```python
from build123d import *

# Parameters (mm, degrees)
SKETCH1_R               = 22.45
BOSS_EXTRUDE1_DEPTH     = 5
SKETCH2_R               = 5
CUT_EXTRUDE1_DEPTH      = 5
BOSS_EXTRUDE2_DEPTH     = 50
BOSS_EXTRUDE5_DEPTH     = 50
CUT_EXTRUDE3_DEPTH      = 64.505944604
CUT_EXTRUDE3_DEPTH_BACK = 64.505944604


with BuildPart() as part:
    # Sketch1 → Boss-Extrude1 (new body)
    with BuildSketch(Plane.XY):
        Circle(SKETCH1_R)
    extrude(amount=BOSS_EXTRUDE1_DEPTH)

    # Sketch2 → Cut-Extrude1 (cut)
    with BuildSketch(Plane(origin=(0, 0, 0), x_dir=(-1, 0, 0), z_dir=(0, 0, -1))):
        Circle(SKETCH2_R)
        with Locations((0, 15)):
            Circle(SKETCH2_R)
    extrude(amount=-CUT_EXTRUDE1_DEPTH, mode=Mode.SUBTRACT)

    # Sketch3 → Boss-Extrude2 (add)
    with BuildSketch(Plane.XY.offset(5)):
        with BuildLine():
            Line((-12.718195627, -18.5), (12.718195627, -18.5))
            ThreePointArc((12.718195627, -18.5), (14.006550731, -17.544772344), (15.223419458, -16.5))
            Line((15.223419458, -16.5), (-15.223419458, -16.5))
            ThreePointArc((-15.223419458, -16.5), (-14.006550731, -17.544772344), (-12.718195627, -18.5))
        make_face()
    extrude(amount=BOSS_EXTRUDE2_DEPTH)

    # Sketch5 → Boss-Extrude5 (add)
    with BuildSketch(Plane.XY.offset(5)):
        with BuildLine():
            Line((-15.223419458, -16.5), (-12.08108025, -16.5))
            ThreePointArc((-12.08108025, -16.5), (-12.994947259, -15.790308602), (-13.867212825, -15.030066815))
            ThreePointArc((-13.867212825, -15.030066815), (-18.732151535, -8.204206169), (-20.45, 0))
            Line((-20.45, 0), (-22.45, 0))
            ThreePointArc((-22.45, 0), (-20.564146795, -9.006573521), (-15.223419458, -16.5))
        make_face()
        with BuildLine():
            Line((20.45, 0), (22.45, 0))
            ThreePointArc((22.45, 0), (20.564146795, -9.006573521), (15.223419458, -16.5))
            Line((15.223419458, -16.5), (12.08108025, -16.5))
            ThreePointArc((12.08108025, -16.5), (12.994947259, -15.790308602), (13.867212825, -15.030066815))
            ThreePointArc((13.867212825, -15.030066815), (18.732151535, -8.204206169), (20.45, 0))
        make_face()
    extrude(amount=BOSS_EXTRUDE5_DEPTH)

    # Sketch6 → Cut-Extrude3 (cut, two sides: drawn at the far end of the back side and taken through both)
    with BuildSketch(Plane(origin=(0, 0, 0), x_dir=(1, 0, 0), z_dir=(0, 1, 0)).offset(-CUT_EXTRUDE3_DEPTH_BACK)):
        Polygon((-22.45, 0), (22.45, 0), (22.45, -2.35310929), align=None)
    extrude(amount=CUT_EXTRUDE3_DEPTH + CUT_EXTRUDE3_DEPTH_BACK, mode=Mode.SUBTRACT)


solid = part.part
```
Source: CAD feature listing. Evaluate the final solid. Frame: model axes, mm. A direction names the side the tool comes from. Give positions to 0.01 mm unless a question says otherwise; leave off trailing zeros. Loops run counter-clockwise (first coordinate to the right, second up) from the corner with the lowest first, then second, coordinate; pieces in that order, holes last. Notation, with made-up numbers: (38, -17.75) - (86, -17.75) arc R9 cw to (86, -10.75) - close; hole circle Ø7 at (2, 34). An arc over 180 degrees is marked (long way). Use CSV: the item, a comma, the result in double quotes. Start each with the question number.
1. Section D-D (y = 4). Output: boundary loops of the cut face in (x, z), then the cut area to 3 significant figures.
2. Reachability of faces 5 (the flat face through (0, -18.5, 30)), 6 (the flat face through (0.314, -5.303, 1.193)), 7 (the flat face through (5, 3, 5)), 8 (the flat face through (-21, 0, 30)) from +Z, -Z, +X, -X, +Y, -Y: full face, straight path, thin tool, end or side. Return the list, or none.
3. Draft query along Y for faces 1 (the flat face through (0, -20, 5)), 2 (the cylindrical face through (-4.619, -1.915, 2.929)), 3 (the flat face through (0, -16.5, 30)), 4 (the cylindrical face through (-4.619, 13.085, 2.929)). Return one class per face: +Y half, -Y half, draft (parallel to the pull), parting line (faces both ways), or undercut.
4. Ray query, L1, parallel to Y at x = 0, z = 3; L2, parallel to X at y = -7, z = 37.5; L3, parallel to X at y = 15, z = 2.5. Return the intervals inside material, ascending.
5. Section C-C (z = 31). Output: boundary loops of the cut face in (x, y), then the cut area to 3 significant figures.
6. Section B-B (x = 3.5). Output: boundary loops of the cut face in (y, z), then the cut area to 3 significant figures.
7. Section A-A (y = -4). Output: boundary loops of the cut face in (x, z).
8. Pin query (flat end, axial travel): pin 1 (3 mm diameter, centred on y = -11.5, z = 14, fed in from -X); pin 2 (3 mm diameter, centred on x = -14, y = 0, fed in from -Z); pin 3 (11.5 mm diameter, centred on x = 0, y = 3.5, fed in from +Z); pin 4 (8 mm diameter, centred on y = 7, z = 35, fed in from -X). Return the tip coordinate at first contact, or that it passes through.
Response:
1,outline,"(-22.09, 0.02) - (-3, 1.02) - (-3, 5) - (-22.09, 5) - close; (3, 1.33) - (22.09, 2.33) - (22.09, 5) - (3, 5) - close"
1,area,"146 mm²"
2,face 5,"+Z, +X, -X, -Y"
2,face 6,"-Z, +X, +Y, -Y"
2,face 7,"+Z, +Y"
2,face 8,"+Z, +X, -X, +Y"
3,face 1,"draft"
3,face 2,"undercut"
3,face 3,"+Y half"
3,face 4,"undercut"
4,L1,"-22.45 to -5, 5 to 10, 20 to 22.45"
4,L2,"-21.33 to -19.21, 19.21 to 21.33"
4,L3,"-16.7 to -5, 5 to 16.7"
5,outline,"(-22.45, 0) arc R22.45 ccw to (-12.72, -18.5) - (12.72, -18.5) arc R22.45 ccw to (22.45, 0) - (20.45, 0) arc R20.45 cw to (12.08, -16.5) - (-12.08, -16.5) arc R20.45 cw to (-20.45, 0) - close"
5,area,"131 mm²"
6,outline,"(-22.18, 1.36) - (-3.57, 1.36) - (-3.57, 5) - (-16.5, 5) - (-16.5, 55) - (-18.5, 55) - (-18.5, 5) - (-22.18, 5) - close; (3.57, 1.36) - (11.43, 1.36) - (11.43, 5) - (3.57, 5) - close; (18.57, 1.36) - (22.18, 1.36) - (22.18, 5) - (18.57, 5) - close"
6,area,"209 mm²"
7,outline,"(-22.09, 0.02) - (-3, 1.02) - (-3, 5) - (-20.05, 5) - (-20.05, 55) - (-22.09, 55) - close; (3, 1.33) - (22.09, 2.33) - (22.09, 55) - (20.05, 55) - (20.05, 5) - (3, 5) - close"
8,pin 1,"x = -20.1"
8,pin 2,"z = 0.36"
8,pin 3,"z = 5"
8,pin 4,"through"
